Here's the drawing with two shaded views (mm, measured from the low corner). I have some questions. Give positions to 0.01 mm unless a question says otherwise; leave off trailing zeros. Write each loop counter-clockwise with the first axis right and the second up, starting at its lowest first coordinate (ties: lowest second). Pieces come first, ordered by that corner, then holes.
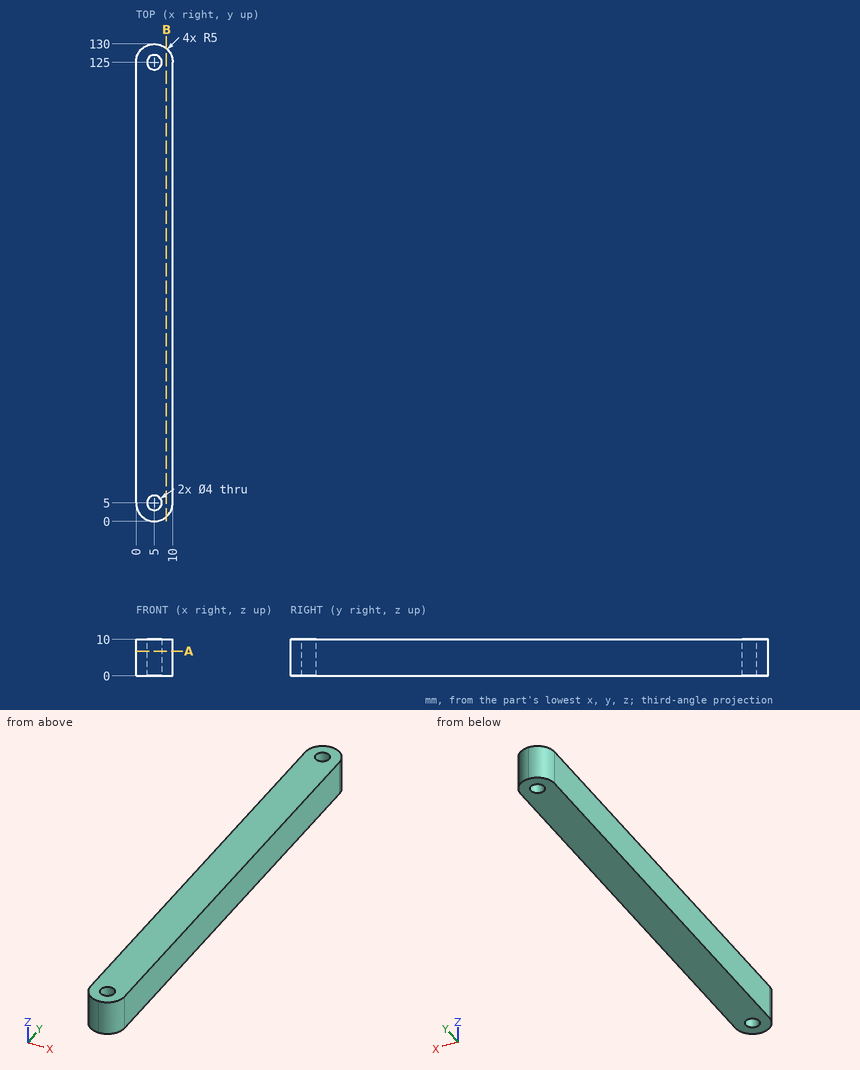
1) Suppose I cut it at A-A on z = 6.75. State how many separate pieces and enclosed holes the cut face has, plus the area to 3 significant figures.
Values follow:
separate pieces: 1
enclosed holes: 2
area: 1,250 mm2
2) Suppose I cut it at B-B on x = 8.25. Write out the boundary of the cut face in (y, z), plus the area to 3 significant figures.
Values follow:
outline: (1.2, 0) - (128.8, 0) - (128.8, 10) - (1.2, 10) - close
area: 1,280 mm2
3) Please list where these lines run through material, in increasing order: L1, parallel to Y at x = 5, z = 6; L2, parallel to Y at x = 6.5, z = 5.5; L3, parallel to Y at x = 1.5, z = 5.5.
Values follow:
L1: y = 0 to 3, 7 to 123, 127 to 130
L2: y = 0.23 to 3.68, 6.32 to 123.68, 126.32 to 129.77
L3: y = 1.43 to 128.57
